Build history of the part. All positions in model axes, mm. Face numbers are marked on the shaded views. Coordinates: 2 decimals unless noted, no trailing zeros. Order: outer loops, then holes, each group sorted by start corner. A loop starts at its lowest first (then second) coordinate and runs counter-clockwise, first axis right, second up. Notation, with made-up numbers: (-36.75, -2.75) -> (-0.75, -2.75) arc R24 cw to (-0.75, 7.25) -> close; hole circle Ø5 at (1, 48.25). An arc over 180 degrees is marked (long way). Write each question's results on one line, items separated by ' | '.
from build123d import *

# Parameters (mm, degrees)
SKETCH1_R           = 16.7
BOSS_EXTRUDE1_DEPTH = 0.4
BOSS_EXTRUDE3_DEPTH = 1
FILLET1_R           = 1


with BuildPart() as part:
    # Sketch1 → Boss-Extrude1 (new body)
    with BuildSketch(Plane(origin=(0, 0, 0), x_dir=(1, 0, 0), z_dir=(0, 1, 0))):
        with BuildLine():
            Line((-7.305730618, 21), (-10.009228055, 15.558449593))
            Line((-10.009228055, 15.558449593), (-10.461777167, 14.647566983))
            ThreePointArc((-10.461777167, 14.647566983), (-13.695076666, 11.68096208), (-16.11449254, 8.020170209))
            Line((-16.11449254, 8.020170209), (-17.457366918, 8.688517726))
            ThreePointArc((-17.457366918, 8.688517726), (-19.248737127, -3.120275469), (-13.818649167, -13.758449593))
            Line((-13.818649167, -13.758449593), (-11.606251109, -13.758449593))
            ThreePointArc((-11.606251109, -13.758449593), (-9.687950737, -15.170484848), (-7.6, -16.316862443))
            Line((-7.6, -16.316862443), (-7.6, -20.407699946))
            Line((-7.6, -20.407699946), (7.6, -20.407699946))
            Line((7.6, -20.407699946), (7.6, -16.316862443))
            ThreePointArc((7.6, -16.316862443), (9.687950737, -15.170484848), (11.606251109, -13.758449593))
            Line((11.606251109, -13.758449593), (13.818649167, -13.758449593))
            ThreePointArc((13.818649167, -13.758449593), (19.248737127, -3.120275469), (17.457366918, 8.688517726))
            Line((17.457366918, 8.688517726), (16.11449254, 8.020170209))
            ThreePointArc((16.11449254, 8.020170209), (13.695076666, 11.68096208), (10.461777167, 14.647566983))
            Line((10.461777167, 14.647566983), (10.009228055, 15.558449593))
            Line((10.009228055, 15.558449593), (7.305730618, 21))
            Line((7.305730618, 21), (-7.305730618, 21))
        make_face()
        with Locations(Location((0, 0, 0), (0, 0, 270))):
            Circle(SKETCH1_R, mode=Mode.SUBTRACT)
    extrude(amount=BOSS_EXTRUDE1_DEPTH)

    # Sketch2 → Boss-Extrude3 (add)
    with BuildSketch(Plane(origin=(0, 0.4, 0), x_dir=(1, 0, 0), z_dir=(0, 1, 0))):
        with BuildLine():
            Line((-8.56095789, 16.4), (-6.705730618, 21))
            Line((-6.705730618, 21), (-7.305730618, 21))
            Line((-7.305730618, 21), (-10.009228055, 15.558449593))
            ThreePointArc((-10.009228055, 15.558449593), (-9.294622278, 15.995624299), (-8.56095789, 16.4))
        make_face()
        with BuildLine():
            Line((8.56095789, 16.4), (6.705730618, 21))
            Line((6.705730618, 21), (7.305730618, 21))
            Line((7.305730618, 21), (10.009228055, 15.558449593))
            ThreePointArc((10.009228055, 15.558449593), (9.294622278, 15.995624299), (8.56095789, 16.4))
        make_face()
        with BuildLine():
            Line((-7.6, -20.407699946), (7.6, -20.407699946))
            Line((7.6, -20.407699946), (7.6, -16.316862443))
            ThreePointArc((7.6, -16.316862443), (0, -18), (-7.6, -16.316862443))
            Line((-7.6, -16.316862443), (-7.6, -20.407699946))
        make_face()
        with BuildLine():
            Line((-16.11449254, 8.020170209), (-17.457366918, 8.688517726))
            ThreePointArc((-17.457366918, 8.688517726), (-19.248737127, -3.120275469), (-13.818649167, -13.758449593))
            Line((-13.818649167, -13.758449593), (-11.606251109, -13.758449593))
            ThreePointArc((-11.606251109, -13.758449593), (-17.626314908, -3.648701519), (-16.11449254, 8.020170209))
        make_face()
        with BuildLine():
            Line((17.457366918, 8.688517726), (16.11449254, 8.020170209))
            ThreePointArc((16.11449254, 8.020170209), (17.626314908, -3.648701519), (11.606251109, -13.758449593))
            Line((11.606251109, -13.758449593), (13.818649167, -13.758449593))
            ThreePointArc((13.818649167, -13.758449593), (19.248737127, -3.120275469), (17.457366918, 8.688517726))
        make_face()
    extrude(amount=BOSS_EXTRUDE3_DEPTH)

    # Fillet1
    fillet1_edges = [part.edges().sort_by_distance(p)[0] for p in [
        (7.6, 0.7, 20.407699946),
        (-7.6, 0.7, 20.407699946),
        (-8.56095789, 0.9, -16.4),
        (8.56095789, 0.9, -16.4),
    ]]
    fillet(fillet1_edges, radius=FILLET1_R)


solid = part.part
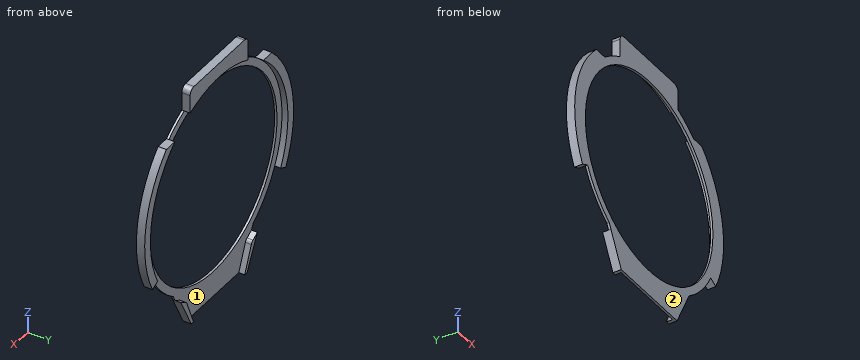
Item 1: Slice it at D-D, the plane z = 7. List the corners of the cut face in (x, y).
Answer:
outline: (-18.2, 0) -> (-15.16, 0) -> (-15.16, 0.4) -> (-16.58, 0.4) -> (-16.58, 1.4) -> (-18.2, 1.4) -> close; (15.16, 0) -> (18.2, 0) -> (18.2, 1.4) -> (16.58, 1.4) -> (16.58, 0.4) -> (15.16, 0.4) -> close
Item 2: Pull direction X, two halves, no side cores. Call the marked faces 1 and 2: released by +X, released by -X, zero draft, split by the parting line, or undercut.
Answer:
face 1: undercut | face 2: zero draft
Item 3: Slice it at C-C, the plane z = 0. List the corners of the cut face in (x, y), and give its area (3 significant figures).
Answer:
outline: (-19.5, 0) -> (-16.7, 0) -> (-16.7, 0.4) -> (-18, 0.4) -> (-18, 1.4) -> (-19.5, 1.4) -> close; (16.7, 0) -> (19.5, 0) -> (19.5, 1.4) -> (18, 1.4) -> (18, 0.4) -> (16.7, 0.4) -> close | area: 5.24 mm^2
Item 4: Drill centre lines: line 1 (X direction, y = 0.15, z = 0); line 2 (X direction, y = 0.35, z = 13); line 3 (Z direction, x = -12.5, y = 0.1). Where is each one in solid material? Low to high. Write a range as from..to.
Answer:
line 1: x = -19.5..-16.7, 16.7..19.5 | line 2: x = -14.53..-10.48, 10.48..14.53 | line 3: z = -12.95..-11.07, 11.07..13.76
Item 5: Slice it at A-A, the plane x = 0. List the corners of the cut face in (y, z).
Answer:
outline: (0, -21) -> (0.4, -21) -> (0.4, -16.7) -> (0, -16.7) -> close; (0, 16.7) -> (0.4, 16.7) -> (0.4, 18) -> (1.4, 18) -> (1.4, 20.41) -> (0, 20.41) -> close
Item 6: Slice it at B-B, the plane y = 1.15. List the corners of the cut face in (x, z), and give its area (3 significant figures).
Answer:
outline: (-17.46, -8.69) -> (-16.11, -8.02) arc R18 cw to (-11.61, 13.76) -> (-13.82, 13.76) arc R19.5 ccw to start; (-10.01, -15.56) -> (-7.31, -21) -> (-6.71, -21) -> (-8.43, -16.74) arc R1 ccw to (-8.87, -16.23) arc R18.5 cw to start; (-7.6, 16.32) arc R18 cw to (7.6, 16.32) -> (7.6, 19.41) arc R1 ccw to (6.6, 20.41) -> (-6.6, 20.41) arc R1 ccw to (-7.6, 19.41) -> close; (6.71, -21) -> (7.31, -21) -> (10.01, -15.56) arc R18.5 cw to (8.87, -16.23) arc R1 ccw to (8.43, -16.74) -> close; (11.61, 13.76) arc R18 cw to (16.11, -8.02) -> (17.46, -8.69) arc R19.5 ccw to (13.82, 13.76) -> close | area: 125 mm^2
